Read the model definition and answer for the solid it produces. Units are mm, in the model's axes. A direction names the side the tool comes from. Give positions to 0.01 mm unless a question says otherwise; leave off trailing zeros. Order: outer loops, then holes, each group sorted by start corner. A loop starts at its lowest first (then second) coordinate and runs counter-clockwise, first axis right, second up.
Item 1: A cutting plane is placed at A-A (z = -2.5). Write down the section's boundary in (x, y), plus the area to 3 significant figures.
Item 2: A cutting plane is placed at C-C (x = 0). Write down the section's boundary in (y, z).
Item 3: A cutting plane is placed at B-B (y = 10.3). State how many separate pieces and enclosed holes the cut face has, plus the area to 3 significant figures.
Item 4: The mould has two halves that part along Y. Classify faces 4 (the face through (-2.95, -10, 7)), 5 (the face through (-13.9, 0, 3)), 6 (the face through (12.15, -10, 10)): +Y half, -Y half, draft (parallel to the pull), parting line (faces both ways), or undercut.
Item 5: Find the intervals of material crossed by line 1 along Y through (x, z) = (9.2, 1); line 2 along X through (y, z) = (2.5, 1); line 3 along X through (y, z) = (0, 3.75), in increasing order.
Item 6: Which of the six approach directions +Z, -Z, +X, -X, +Y, -Y give full straight-line access (tool end or side, diameter ignored) to faces 1 (the face through (0, 13.25, 7)), 2 (the face through (-10, -3.1, 4)), 3 (the face through (4.1, -5, -10))?
Item 7: Given pin 1 Ø1.9 at (y, z) = (-1, 1) entering from -X; pin 2 Ø1.9 at (y, z) = (12.5, -10) entering from -X; pin 3 Ø0.8 at (y, z) = (-4, -10) entering from +X, each flat-ended and moving along its own axis, determine where each tip first touches the part or whether it passes through.
from build123d import *

# Parameters (mm, degrees)
SKETCH2_W               = 27.8
SKETCH2_H               = 18
SKETCH2_R               = 6
BOSS_EXTRUDE1_DEPTH     = 15
SKETCH7_W               = 13.9
SKETCH7_H               = 15
SKETCH7_W_2             = 5.9
SKETCH7_H_2             = 5.9
BOSS_EXTRUDE3_DEPTH     = 1.8
SKETCH8_R               = 1.7
CUT_EXTRUDE3_DEPTH      = 29.464890655
FILLET4_R               = 0.5
FILLET4_OF_MIRROR1_R    = 0.5
MIRROR2_START           = -9
MIRROR2_OUTLINE_R       = 1.7
MIRROR2_DEPTH           = 18
MIRROR2_START_2         = 9
MIRROR2_2_OUTLINE_W     = 13.9
MIRROR2_2_OUTLINE_H     = 30
MIRROR2_2_DEPTH         = 1.8
FILLET3_R               = 2
BOSS_EXTRUDE4_DEPTH     = 1.7
CUT_EXTRUDE4_REACH      = 33.173
CUT_EXTRUDE4_END_RADIUS = 6
CUT_EXTRUDE4_START      = -1.5
SKETCH10_W              = 5.9
SKETCH10_H              = 5.9
FILLET5_R               = 0.5
SKETCH11_R              = 1.7
CUT_EXTRUDE5_DEPTH      = 29.604370348
FILLET5_OF_MIRROR3_R    = 0.5
CUT_EXTRUDE6_START      = -10.8
SKETCH12_W              = 2.2
SKETCH12_H              = 6.2
CUT_EXTRUDE6_DEPTH      = 10.8
SKETCH13_W              = 2.2
SKETCH13_H              = 6.2
CUT_EXTRUDE7_DEPTH      = 2.95
CUT_EXTRUDE8_REACH      = 35.384
CUT_EXTRUDE8_END_RADIUS = 6
SKETCH14_R              = 1.7


# Read off the part's stored shape, not the designer's step: Mirror2
with BuildPart() as part:
    # Sketch2 → Boss-Extrude1 (new, symmetric)
    with BuildSketch(Plane(origin=(0, 0, 0), x_dir=(1, 0, 0), z_dir=(0, 1, 0))):
        Rectangle(SKETCH2_W, SKETCH2_H)
        with Locations(Location((0, 0, 0), (0, 0, 270))):
            Circle(SKETCH2_R, mode=Mode.SUBTRACT)
    extrude(amount=BOSS_EXTRUDE1_DEPTH, both=True)

    # Sketch7 → Boss-Extrude3 (add)
    with BuildSketch(Plane.XY.offset(9)):
        with Locations((-6.95, 7.5)):
            Rectangle(SKETCH7_W, SKETCH7_H)
        with Locations((-9.2, 10.3)):
            Rectangle(SKETCH7_W_2, SKETCH7_H_2, mode=Mode.SUBTRACT)
    boss_extrude3 = extrude(amount=BOSS_EXTRUDE3_DEPTH)

    # Sketch8 → Cut-Extrude3 (cut, through all)
    with BuildSketch(Plane.XY.offset(10.8)):
        with Locations((-9.2, 10.3)):
            Circle(SKETCH8_R)
    cut_extrude3 = extrude(amount=-CUT_EXTRUDE3_DEPTH, mode=Mode.SUBTRACT)

    # Fillet4
    fillet4_edges = [part.edges().sort_by_distance(p)[0] for p in [
        (-6.25, 13.25, 9.9),
        (-12.15, 13.25, 9.9),
        (-12.15, 7.35, 9.9),
        (-6.25, 7.35, 9.9),
    ]]
    fillet(fillet4_edges, radius=FILLET4_R)

    # Mirror1: Boss-Extrude3, Cut-Extrude3 across plane
    add(boss_extrude3.mirror(Plane.ZX))
    add(cut_extrude3.mirror(Plane.ZX), mode=Mode.SUBTRACT)

    # Fillet4 of Mirror1
    fillet4_of_mirror1_edges = [part.edges().sort_by_distance(p)[0] for p in [
        (-6.25, -13.25, 9.9),
        (-12.15, -13.25, 9.9),
        (-12.15, -7.35, 9.9),
        (-6.25, -7.35, 9.9),
    ]]
    fillet(fillet4_of_mirror1_edges, radius=FILLET4_OF_MIRROR1_R)

    # Mirror2 outline → Mirror2 (cut)
    with BuildSketch(Plane.XY.offset(MIRROR2_START)):
        with Locations((9.2, -10.3)):
            Circle(MIRROR2_OUTLINE_R)
        with Locations((9.2, 10.3)):
            Circle(MIRROR2_OUTLINE_R)
    extrude(amount=MIRROR2_DEPTH, mode=Mode.SUBTRACT)

    # Mirror2 2 outline → Mirror2 2 (add)
    with BuildSketch(Plane.XY.offset(MIRROR2_START_2)):
        with Locations((6.95, 0)):
            Rectangle(MIRROR2_2_OUTLINE_W, MIRROR2_2_OUTLINE_H)
        with BuildLine():
            ThreePointArc((6.25, -7.85), (6.396446609, -7.496446609), (6.75, -7.35))
            Line((6.75, -7.35), (11.65, -7.35))
            ThreePointArc((11.65, -7.35), (12.003553391, -7.496446609), (12.15, -7.85))
            Line((12.15, -7.85), (12.15, -12.75))
            ThreePointArc((12.15, -12.75), (12.003553391, -13.103553391), (11.65, -13.25))
            Line((11.65, -13.25), (6.75, -13.25))
            ThreePointArc((6.75, -13.25), (6.396446609, -13.103553391), (6.25, -12.75))
            Line((6.25, -12.75), (6.25, -7.85))
        make_face(mode=Mode.SUBTRACT)
        with BuildLine():
            Line((6.75, 13.25), (11.65, 13.25))
            ThreePointArc((11.65, 13.25), (12.003553391, 13.103553391), (12.15, 12.75))
            Line((12.15, 12.75), (12.15, 7.85))
            ThreePointArc((12.15, 7.85), (12.003553391, 7.496446609), (11.65, 7.35))
            Line((11.65, 7.35), (6.75, 7.35))
            ThreePointArc((6.75, 7.35), (6.396446609, 7.496446609), (6.25, 7.85))
            Line((6.25, 7.85), (6.25, 12.75))
            ThreePointArc((6.25, 12.75), (6.396446609, 13.103553391), (6.75, 13.25))
        make_face(mode=Mode.SUBTRACT)
    extrude(amount=MIRROR2_2_DEPTH)

    # Fillet3
    fillet3_edges = [part.edges().sort_by_distance(p)[0] for p in [
        (-13.9, 15, 0.9),
        (13.9, 15, 0.9),
        (-13.9, -15, 0.9),
        (13.9, -15, 0.9),
    ]]
    fillet(fillet3_edges, radius=FILLET3_R)

    # Sketch9 → Boss-Extrude4 (add)
    with BuildSketch(Plane(origin=(0, 0, -9), x_dir=(-1, 0, 0), z_dir=(0, 0, -1))):
        Polygon((-3.1, 15), (3.1, 15), (3.1, 6), (4.1, 6), (4.1, -15), (-4.1, -15), (-4.1, 6), (-3.1, 6), align=None)
    extrude(amount=BOSS_EXTRUDE4_DEPTH)

    # Cut-Extrude4: up to this cylinder (the profile starts outside it)
    cut_extrude4_end = Plane(origin=(0, 10.3, 0), z_dir=(0, -1, 0)) * Cylinder(CUT_EXTRUDE4_END_RADIUS, 79.346, mode=Mode.PRIVATE)
    # Sketch10 → Cut-Extrude4 (cut, up to the surface)
    with BuildSketch(Plane.XY.offset(10.8).offset(CUT_EXTRUDE4_START), mode=Mode.PRIVATE) as cut_extrude4_sk1:
        with Locations((0, 10.3)):
            Rectangle(SKETCH10_W, SKETCH10_H)
    cut_extrude4_tool1 = extrude(cut_extrude4_sk1.sketch, amount=-CUT_EXTRUDE4_REACH, mode=Mode.PRIVATE) - cut_extrude4_end
    cut_extrude4 = cut_extrude4_tool1.solids().sort_by_distance((0, 10.3, 9.3))[0]
    add(cut_extrude4, mode=Mode.SUBTRACT)

    # Fillet5
    fillet5_edges = [part.edges().sort_by_distance(p)[0] for p in [
        (2.95, 13.25, 7.262350474),
        (2.95, 7.35, 7.262350474),
        (-2.95, 7.35, 7.262350474),
        (-2.95, 13.25, 7.262350474),
    ]]
    fillet(fillet5_edges, radius=FILLET5_R)

    # Sketch11 → Cut-Extrude5 (cut, through all)
    with BuildSketch(Plane(origin=(0, 0, 9.3), x_dir=(-1, 0, 0), z_dir=(0, 0, -1))):
        with Locations((0, 10.3)):
            Circle(SKETCH11_R)
    cut_extrude5 = extrude(amount=-CUT_EXTRUDE5_DEPTH, mode=Mode.SUBTRACT)

    # Mirror3: Cut-Extrude4, Cut-Extrude5 across plane
    add(cut_extrude4.mirror(Plane.ZX), mode=Mode.SUBTRACT)
    add(cut_extrude5.mirror(Plane.ZX), mode=Mode.SUBTRACT)

    # Fillet5 of Mirror3
    fillet5_of_mirror3_edges = [part.edges().sort_by_distance(p)[0] for p in [
        (2.95, -13.25, 7.262350474),
        (2.95, -7.35, 7.262350474),
        (-2.95, -7.35, 7.262350474),
        (-2.95, -13.25, 7.262350474),
    ]]
    fillet(fillet5_of_mirror3_edges, radius=FILLET5_OF_MIRROR3_R)

    # Sketch12 → Cut-Extrude6 (cut)
    with BuildSketch(Plane.XY.offset(10.8).offset(CUT_EXTRUDE6_START)):
        with Locations((-9.8, 0)):
            Rectangle(SKETCH12_W, SKETCH12_H)
    cut_extrude6 = extrude(amount=CUT_EXTRUDE6_DEPTH, mode=Mode.SUBTRACT)

    # Sketch13 → Cut-Extrude7 (cut)
    with BuildSketch(Plane.XY):
        with Locations((-9.8, 0)):
            Rectangle(SKETCH13_W, SKETCH13_H)
    cut_extrude7 = extrude(amount=-CUT_EXTRUDE7_DEPTH, mode=Mode.SUBTRACT)

    # Cut-Extrude8: up to this cylinder (the profile starts outside it)
    cut_extrude8_end = Plane(origin=(0, 0, 0), z_dir=(0, -1, 0)) * Cylinder(CUT_EXTRUDE8_END_RADIUS, 83.768, mode=Mode.PRIVATE)
    # Sketch14 → Cut-Extrude8 (cut, up to the surface)
    with BuildSketch(Plane.ZY.offset(13.9), mode=Mode.PRIVATE) as cut_extrude8_sk1:
        Circle(SKETCH14_R)
    cut_extrude8_tool1 = extrude(cut_extrude8_sk1.sketch, amount=-CUT_EXTRUDE8_REACH, mode=Mode.PRIVATE) - cut_extrude8_end
    cut_extrude8 = cut_extrude8_tool1.solids().sort_by_distance((-13.9, 0, 0))[0]
    add(cut_extrude8, mode=Mode.SUBTRACT)

    # Mirror4: Cut-Extrude6, Cut-Extrude7, Cut-Extrude8 across plane
    add(cut_extrude6.mirror(Plane(origin=(0, 0, 0), x_dir=(0, 0, 1), z_dir=(1, 0, 0))), mode=Mode.SUBTRACT)
    add(cut_extrude7.mirror(Plane(origin=(0, 0, 0), x_dir=(0, 0, 1), z_dir=(1, 0, 0))), mode=Mode.SUBTRACT)
    add(cut_extrude8.mirror(Plane(origin=(0, 0, 0), x_dir=(0, 0, 1), z_dir=(1, 0, 0))), mode=Mode.SUBTRACT)


solid = part.part
Response values:
1. outline: (-13.9, -13) arc R2 ccw to (-11.9, -15) - (-5.45, -15) - (-5.45, 15) - (-11.9, 15) arc R2 ccw to (-13.9, 13) - close; (5.45, -15) - (11.9, -15) arc R2 ccw to (13.9, -13) - (13.9, 13) arc R2 ccw to (11.9, 15) - (5.45, 15) - close; hole circle Ø3.4 at (-9.2, -10.3); hole (-10.9, -3.1) - (-8.7, -3.1) - (-8.7, 3.1) - (-10.9, 3.1) - close; hole circle Ø3.4 at (-9.2, 10.3); hole circle Ø3.4 at (9.2, -10.3); hole circle Ø3.4 at (9.2, 10.3); hole (8.7, -3.1) - (10.9, -3.1) - (10.9, 3.1) - (8.7, 3.1) - close
1. area: 440 mm2
2. outline: (-15, -10.7) - (15, -10.7) - (15, -6) - (-15, -6) - close; (-15, 6) - (-13.25, 6) - (-13.25, 9.3) - (-12, 9.3) - (-12, 10.8) - (-15, 10.8) - close; (-8.6, 9.3) - (-7.35, 9.3) - (-7.35, 6) - (7.35, 6) - (7.35, 9.3) - (8.6, 9.3) - (8.6, 10.8) - (-8.6, 10.8) - close; (12, 9.3) - (13.25, 9.3) - (13.25, 6) - (15, 6) - (15, 10.8) - (12, 10.8) - close
3. separate pieces: 3
3. enclosed holes: 0
3. area: 278 mm2
4. face 4: undercut
4. face 5: draft
4. face 6: undercut
5. line 1: y = -15 to -12, -8.6 to -3.1, 3.1 to 8.6, 12 to 15
5. line 2: x = -13.9 to -10.9, -8.7 to -5.92, 5.92 to 8.7, 10.9 to 13.9
5. line 3: x = -13.9 to -10.9, -8.7 to -4.68, 4.68 to 8.7, 10.9 to 13.9
6. face 1: none
6. face 2: +Z
6. face 3: -Z, +X, +Y, -Y
7. pin 1: stops at x = -13.9
7. pin 2: stops at x = -3.1
7. pin 3: stops at x = 4.1
